Geometry check sheet. Reference: the model listing, model coordinates, mm. Face numbers are marked on the shaded views. Give positions to 0.01 mm unless a question says otherwise; leave off trailing zeros. Loops run counter-clockwise (first coordinate to the right, second up) from the corner with the lowest first, then second, coordinate; pieces in that order, holes last. Notation, with made-up numbers: (-31, -29.5) -> (-25, -29.5) arc R18 ccw to (-25, -0.5) -> close; hole circle Ø7 at (8, -11). An arc over 180 degrees is marked (long way). One line per item, written item: value. Start each with the question number.
(1) Gauge pin test, flat ends, axial feed: pin 1 Ø5 at (y, z) = (2, -5.5) entering from -X; pin 2 Ø3 at (y, z) = (6.5, -10) entering from -X; pin 3 Ø11.5 at (x, z) = (0, 0) entering from -Y. Record the tip position at first contact, or that the pin passes through.
(2) Sectioned sample at A-A, the plane y = 8.5. Record the cut outline in (x, z), then the cut area to 3 significant figures.
(3) Sectioned sample at B-B, the plane z = 5.6. Record the cut outline in (x, y).
(4) Scan lines: line 1 along X through (y, z) = (7.5, 4.75); line 2 along X through (y, z) = (2.5, 5.6); line 3 along Z through (x, y) = (-5.75, 1.75). Record each from-to range of solid material in increasing order. Write a range as from..to.
(5) Sectioned sample at D-D, the plane x = 0.75. Record the cut outline in (y, z), then the cut area to 3 significant figures.
(6) Sectioned sample at C-C, the plane x = 4.25. Record the cut outline in (y, z), then the cut area to 3 significant figures.
(7) Draft check along Z on the marked faces 1, 2, 3 and 4. Enter one of: pulls with the +Z half, pulls with the -Z half, needs draft (parallel to the pull), parting line crosses it, or undercut.
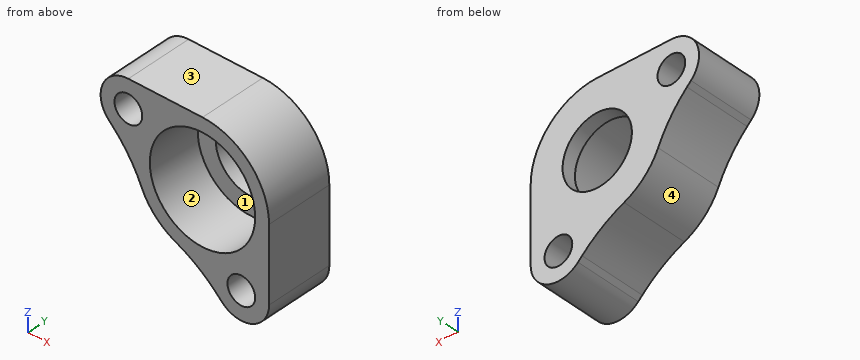
from build123d import *

# Parameters (mm, degrees)
SKETCH1_R           = 2
SKETCH1_R_2         = 7.6
BOSS_EXTRUDE1_DEPTH = 7.75
SKETCH2_R           = 2
SKETCH2_R_2         = 5
BOSS_EXTRUDE2_DEPTH = 2
FILLET1_R           = 20


with BuildPart() as part:
    # Sketch1 → Boss-Extrude1 (new body)
    with BuildSketch(Plane(origin=(0, 0, 0), x_dir=(1, 0, 0), z_dir=(0, 1, 0))):
        with BuildLine():
            Line((2.771572875, 13.519595949), (-1.226723266, 9.521299808))
            ThreePointArc((-1.226723266, 9.521299808), (-6.788225099, 6.788225099), (-9.521299808, 1.226723266))
            Line((-9.521299808, 1.226723266), (-13.519595949, -2.771572875))
            ThreePointArc((-13.519595949, -2.771572875), (-14.386686955, -7.130733729), (-10.691168825, -9.6))
            Line((-10.691168825, -9.6), (0, -9.6))
            ThreePointArc((0, -9.6), (6.788225099, -6.788225099), (9.6, 0))
            Line((9.6, 0), (9.6, 10.691168825))
            ThreePointArc((9.6, 10.691168825), (7.130733729, 14.386686955), (2.771572875, 13.519595949))
        make_face()
        with Locations(Location((-10.691168825, -5.6, 0), (0, 0, 270))):
            Circle(SKETCH1_R, mode=Mode.SUBTRACT)
        with Locations(Location((0, 0, 0), (0, 0, 270))):
            Circle(SKETCH1_R_2, mode=Mode.SUBTRACT)
        with Locations(Location((5.6, 10.691168825, 0), (0, 0, 270))):
            Circle(SKETCH1_R, mode=Mode.SUBTRACT)
    extrude(amount=BOSS_EXTRUDE1_DEPTH)

    # Sketch2 → Boss-Extrude2 (add)
    with BuildSketch(Plane(origin=(0, 7.75, 0), x_dir=(1, 0, 0), z_dir=(0, 1, 0))):
        with BuildLine():
            Line((9.6, 0), (9.6, 10.691168825))
            ThreePointArc((9.6, 10.691168825), (7.130733729, 14.386686955), (2.771572875, 13.519595949))
            Line((2.771572875, 13.519595949), (-1.226723266, 9.521299808))
            ThreePointArc((-1.226723266, 9.521299808), (-6.788225099, 6.788225099), (-9.521299808, 1.226723266))
            Line((-9.521299808, 1.226723266), (-13.519595949, -2.771572875))
            ThreePointArc((-13.519595949, -2.771572875), (-14.386686955, -7.130733729), (-10.691168825, -9.6))
            Line((-10.691168825, -9.6), (0, -9.6))
            ThreePointArc((0, -9.6), (6.788225099, -6.788225099), (9.6, 0))
        make_face()
        with Locations(Location((-10.691168825, -5.6, 0), (0, 0, 270))):
            Circle(SKETCH2_R, mode=Mode.SUBTRACT)
        with Locations(Location((5.6, 10.691168825, 0), (0, 0, 270))):
            Circle(SKETCH2_R, mode=Mode.SUBTRACT)
        with Locations(Location((0, 0, 0), (0, 0, 270))):
            Circle(SKETCH2_R_2, mode=Mode.SUBTRACT)
    extrude(amount=BOSS_EXTRUDE2_DEPTH)

    # Fillet1
    fillet1_edges = [part.edges().sort_by_distance(p)[0] for p in [
        (-9.521299808, 4.875, -1.226723266),
        (-1.226723266, 4.875, -9.521299808),
    ]]
    fillet(fillet1_edges, radius=FILLET1_R)


solid = part.part
Calculated:
1. pin 1: stops at x = -9.2
1. pin 2: stops at x = -4.46
1. pin 3: stops at y = 7.75
2. outline: (-13.52, 2.77) -> (-12.94, 2.19) arc R20 cw to (-8.78, -3.88) arc R9.6 ccw to (-3.88, -8.78) arc R20 cw to (2.19, -12.94) -> (2.77, -13.52) arc R4 ccw to (9.6, -10.69) -> (9.6, 0) arc R9.6 ccw to (0, 9.6) -> (-10.69, 9.6) arc R4 ccw to start; hole circle Ø4 at (-10.69, 5.6); hole circle Ø10 at (0, 0); hole circle Ø4 at (5.6, -10.69)
2. area: 304 mm2
3. outline: (-14.69, 0) -> (-12.69, 0) -> (-12.69, 9.75) -> (-14.69, 9.75) -> close; (-8.69, 0) -> (-5.14, 0) -> (-5.14, 7.75) -> (5.14, 7.75) -> (5.14, 0) -> (7.8, 0) -> (7.8, 9.75) -> (-8.69, 9.75) -> close
4. line 1: x = -14.6..-12.5, -8.88..-5.93, 5.93..8.34
4. line 2: x = -14.69..-12.69, -8.69..-5.14, 5.14..7.8
4. line 3: z = -7.69..-4.97, 4.97..9.6
5. outline: (0, -11.63) -> (9.75, -11.63) -> (9.75, -4.94) -> (7.75, -4.94) -> (7.75, -7.56) -> (0, -7.56) -> close; (0, 7.56) -> (7.75, 7.56) -> (7.75, 4.94) -> (9.75, 4.94) -> (9.75, 9.57) -> (0, 9.57) -> close
5. area: 69.7 mm2
6. outline: (0, -14.46) -> (9.75, -14.46) -> (9.75, -12.17) -> (0, -12.17) -> close; (0, -9.22) -> (9.75, -9.22) -> (9.75, -2.63) -> (7.75, -2.63) -> (7.75, -6.3) -> (0, -6.3) -> close; (0, 6.3) -> (7.75, 6.3) -> (7.75, 2.63) -> (9.75, 2.63) -> (9.75, 8.61) -> (0, 8.61) -> close
6. area: 87.9 mm2
7. face 1: undercut
7. face 2: undercut
7. face 3: pulls with the +Z half
7. face 4: pulls with the -Z half
